Can you work these out from the model? Positions are in its coordinate system, mm. Face numbers are marked on the shaded views. A direction names the side the tool comes from. Round coordinates to 2 decimals unless told otherwise and drop trailing zeros. Write each loop counter-clockwise with the first axis right and the second up, starting at its lowest first coordinate (ties: lowest second). Pieces come first, ordered by that corner, then holes.
Q1. If we section it at B-B (z = 15.25): Please give me the cut outline in (x, y), plus the area to 3 significant figures.
Q2. I'm going to push flat-ended pins straight in: pin 1 Ø0.6 at (y, z) = (-7.5, 7.5) entering from +X; pin 2 Ø1.5 at (y, z) = (7.5, 6) entering from +X; pin 3 Ø1.2 at (x, z) = (-7, 9.5) entering from -Y. Where does each tip first touch, or does it pass through?
Q3. If we section it at A-A (y = 0): Please give me the cut outline in (x, z).
Q4. If we section it at C-C (x = -16): Please give me the cut outline in (y, z).
Q5. For the marked faces 4 and 5, which set-ups out of +Z, -Z, +X, -X, +Y, -Y let a thin tool reach every point of the face, with its end or its side?
Q6. We'd pull the mould along Y, two halves only. Please class the marked faces 1, 2 and 3: +Y half, -Y half, draft (parallel to the pull), parting line (faces both ways), or undercut.
Q7. If we section it at D-D (y = -5.25): Please give me the cut outline in (x, z), plus the area to 3 significant figures.
Q8. Please list where these lines run through material, in increasing order: line 1 along X through (y, z) = (-3.25, 1); line 2 along X through (y, z) = (0.5, 5.25); line 3 along Y through (x, z) = (13, 13).
from build123d import *

# Parameters (mm, degrees)
F0_R     = 2.75
F1_DEPTH = 20


with BuildPart() as f1:
    # F0 (on Top) → F1 (new body)
    with BuildSketch(Plane.XY):
        with BuildLine():
            Line((25.054192, 6.176512), (20.054192, 11.176512))
            Line((20.054192, 11.176512), (-19.945808, 11.176512))
            Line((-19.945808, 11.176512), (-24.945808, 6.176512))
            ThreePointArc((-24.945808, 6.176512), (-16.851883, -8.388866), (-1.224984, -14.173488))
            Line((-1.224984, -14.173488), (1.333368, -14.173488))
            ThreePointArc((1.333368, -14.173488), (16.960268, -8.388866), (25.054192, 6.176512))
        make_face()
        with Locations((-14.560476, -1.173488)):
            Circle(F0_R, mode=Mode.SUBTRACT)
        with BuildLine():
            Line((5.694343, 2.05741), (8.054192, 2.05741))
            Line((8.054192, 2.05741), (8.054192, -3.94259))
            Line((8.054192, -3.94259), (5.934845, -3.94259))
            ThreePointArc((5.934845, -3.94259), (4.847493, -5.563735), (3.327843, -6.788932))
            Line((3.327843, -6.788932), (3.327843, -9.173488))
            Line((3.327843, -9.173488), (-2.672157, -9.173488))
            Line((-2.672157, -9.173488), (-2.672157, -7.074083))
            ThreePointArc((-2.672157, -7.074083), (-4.525293, -5.786331), (-5.82646, -3.94259))
            Line((-5.82646, -3.94259), (-7.945808, -3.94259))
            Line((-7.945808, -3.94259), (-7.945808, 2.05741))
            Line((-7.945808, 2.05741), (-5.585958, 2.05741))
            ThreePointArc((-5.585958, 2.05741), (-4.336867, 3.619069), (-2.672157, 4.727107))
            Line((-2.672157, 4.727107), (-2.672157, 6.826512))
            Line((-2.672157, 6.826512), (3.327843, 6.826512))
            Line((3.327843, 6.826512), (3.327843, 4.441956))
            ThreePointArc((3.327843, 4.441956), (4.667811, 3.405215), (5.694343, 2.05741))
        make_face(mode=Mode.SUBTRACT)
        with Locations((14.668861, -1.173488)):
            Circle(F0_R, mode=Mode.SUBTRACT)
    extrude(amount=F1_DEPTH)


solid = f1.part
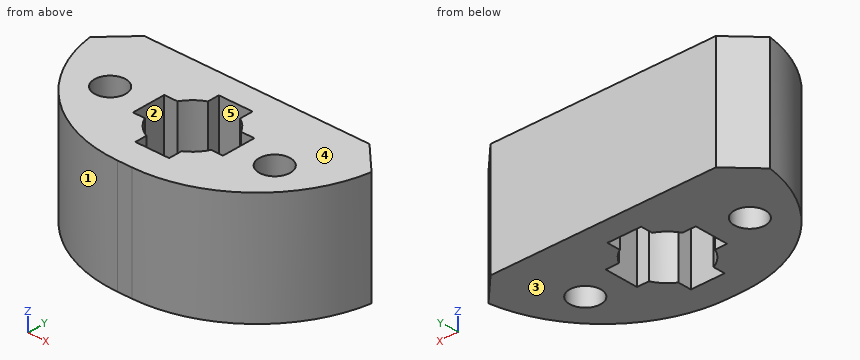
A:
1. outline: (-24.95, 6.18) arc R24 ccw to (-1.22, -14.17) - (1.33, -14.17) arc R24 ccw to (25.05, 6.18) - (20.05, 11.18) - (-19.95, 11.18) - close; hole circle Ø5.5 at (-14.56, -1.17); hole (-7.95, -3.94) - (-5.83, -3.94) arc R6.5 ccw to (-2.67, -7.07) - (-2.67, -9.17) - (3.33, -9.17) - (3.33, -6.79) arc R6.5 ccw to (5.93, -3.94) - (8.05, -3.94) - (8.05, 2.06) - (5.69, 2.06) arc R6.5 ccw to (3.33, 4.44) - (3.33, 6.83) - (-2.67, 6.83) - (-2.67, 4.73) arc R6.5 ccw to (-5.59, 2.06) - (-7.95, 2.06) - close; hole circle Ø5.5 at (14.67, -1.17)
1. area: 785 mm2
2. pin 1: stops at x = 18.25
2. pin 2: stops at x = 24.48
2. pin 3: stops at y = -13.61
3. outline: (-23.12, 0) - (-17.05, 0) - (-17.05, 20) - (-23.12, 20) - close; (-12.07, 0) - (-7.95, 0) - (-7.95, 20) - (-12.07, 20) - close; (8.05, 0) - (12.18, 0) - (12.18, 20) - (8.05, 20) - close; (17.16, 0) - (23.23, 0) - (23.23, 20) - (17.16, 20) - close
4. outline: (-9.09, 0) - (-3.52, 0) - (-3.52, 20) - (-9.09, 20) - close; (1.17, 0) - (11.18, 0) - (11.18, 20) - (1.17, 20) - close
5. face 4: +Z, +X, -X, +Y, -Y
5. face 5: +Z, -Z
6. face 1: -Y half
6. face 2: undercut
6. face 3: draft
7. outline: (-19.9, 0) - (-5.01, 0) - (-5.01, 20) - (-19.9, 20) - close; (5.12, 0) - (20.01, 0) - (20.01, 20) - (5.12, 20) - close
7. area: 596 mm2
8. line 1: x = -21.35 to -16.36, -12.76 to -7.95, 8.05 to 12.87, 16.47 to 21.46
8. line 2: x = -23.34 to -16.74, -12.38 to -7.95, 8.05 to 12.49, 16.85 to 23.45
8. line 3: y = -11.15 to -3.36, 1.01 to 11.18
